Autodesk Inventor part; units mm, degrees
ref_plane "YZ Plane" through (0, 0, 0) normal (1, 0, 0) x (0, 1, 0)
ref_plane "XZ Plane" through (0, 0, 0) normal (0, 1, 0) x (-1, 0, 0)
ref_plane "XY Plane" through (0, 0, 0) normal (0, 0, 1) x (1, 0, 0)
sketch "Sketch1" plane through (0, 0, 0) normal (0, 1, 0) x (-1, 0, 0)
  line L0 (0, 0) -> (203.2, 0)
  line L1 (203.2, 0) -> (203.2, -203.2)
  line L2 (203.2, -203.2) -> (0, -203.2)
  line L3 (0, -203.2) -> (0, 0)
  circle A0 centre (101.6, -101.6) radius 19.05
  dimension "d0" = 203.2
  dimension "d1" = 203.2
  dimension "d4" = 38.1
  dimension "d5" = 101.6
  dimension "d6" = 101.6
extrude "Extrusion1" add sketch "Sketch1" along normal blind 6.35
properties part number "Plate8inx8in"
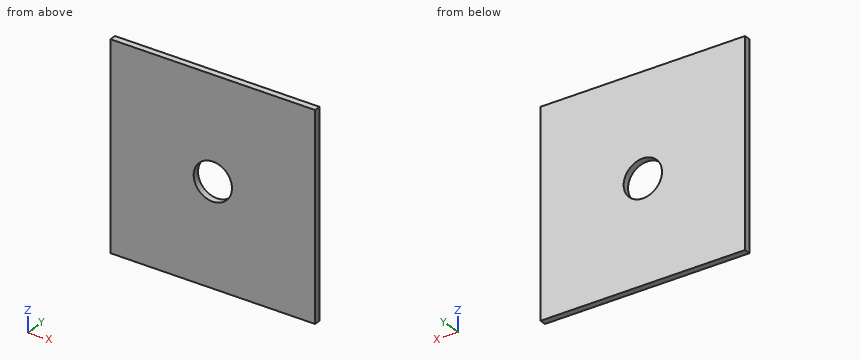
Source: CAD feature listing. Evaluate the final solid. Frame: model axes, mm. Coordinates: 2 decimals unless noted, no trailing zeros. Loops run counter-clockwise (first coordinate to the right, second up) from the corner with the lowest first, then second, coordinate; pieces in that order, holes last. Notation, with made-up numbers: (82, 43) - (128, 43) arc R30 ccw to (128, 70) - close; hole circle Ø6 at (72.25, 11). An arc over 180 degrees is marked (long way). One line per item, written item: value. Start each with the question number.
1. Ray query, L1, parallel to Z at x = -101.6, y = 4; L2, parallel to X at y = 2.75, z = -95; L3, parallel to X at y = 2.25, z = -98.5. Return the intervals inside material, ascending.
2. Section C-C (y = 1.75). Return the cut outline in (x, z), and give its area (3 significant figures).
3. Section B-B (z = -101.6). Return the cut outline in (x, y).
4. Contact query for a flat-ended pin moving along its axis: P1, Ø1, axis at x = -106.5, y = 4.5, coming from the +Z side. Output: stop coordinate, or through.
5. Section A-A (x = -101.6). Return the cut outline in (y, z), and give its area (3 significant figures).
Verdict:
1. L1: z = -203.2 to -120.65, -82.55 to 0
1. L2: x = -203.2 to -119.47, -83.73 to 0
1. L3: x = -203.2 to -120.4, -82.8 to 0
2. outline: (-203.2, -203.2) - (0, -203.2) - (0, 0) - (-203.2, 0) - close; hole circle Ø38.1 at (-101.6, -101.6)
2. area: 40,200 mm2
3. outline: (-203.2, 0) - (-120.65, 0) - (-120.65, 6.35) - (-203.2, 6.35) - close; (-82.55, 0) - (0, 0) - (0, 6.35) - (-82.55, 6.35) - close
4. P1: stops at z = 0
5. outline: (0, -203.2) - (6.35, -203.2) - (6.35, -120.65) - (0, -120.65) - close; (0, -82.55) - (6.35, -82.55) - (6.35, 0) - (0, 0) - close
5. area: 1,050 mm2
